The model under review builds one solid part; all positions refer to its coordinate system, in mm. Face numbers are marked on the shaded views. A direction names the side the tool comes from. Round coordinates to 2 decimals unless told otherwise and drop trailing zeros. Loops run counter-clockwise (first coordinate to the right, second up) from the corner with the lowest first, then second, coordinate; pieces in that order, holes last. Notation, with made-up numbers: M 1,79.5 L 27,79.5 A17 ccw 27,111.5 Z; hole C 87.25,20 d1. An arc over 180 degrees is marked long. Answer as a JSON object with one key per item and string values. Group by question number.
Item 1: Consider section A-A (x = 9.25). Give the boundary of the cut face in (y, z).
Item 2: Insertion check: P1, Ø0.5, axis at x = -3.5, z = -0.5, coming from the +Y side; P2, Ø1, axis at x = 11, z = 3, coming from the -Y side; P3, Ø2, axis at x = 1.5, z = -0.5, coming from the +Y side. Each pin has a flat end and moves straight along its axis. Give the tip position at first contact, or say it passes through.
Item 3: Tool access review of the marked faces 1 and 2: name each direction out of +Z, -Z, +X, -X, +Y, -Y from which nothing blocks a thin tool from reaching the whole face with its end or side.
Item 4: The part is to be moulded in two halves that separate along Z. For the marked faces 3 and 4, say which applies: +Z half, -Z half, draft (parallel to the pull), parting line (faces both ways), or undercut.
Item 5: To check wall thickness, follow line 1 (X direction, y = 1, z = 4.25); line 2 (X direction, y = 1.25, z = 1.75); line 3 (X direction, y = 2, z = -0.25). State the ranges of each line that lie inside material, in increasing order.
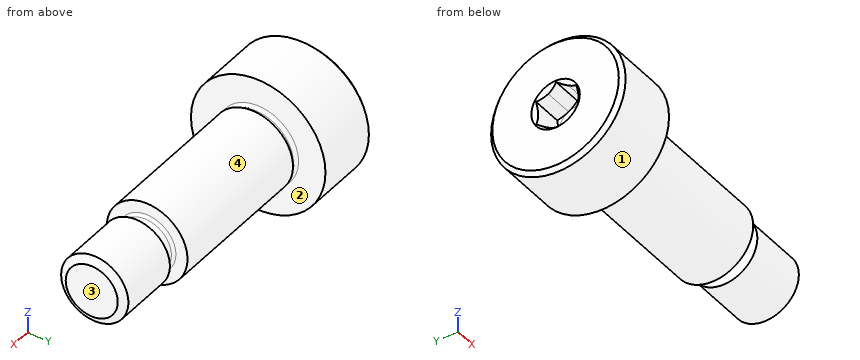
```python
from build123d import *

# Parameters (mm, degrees)
HEXEXTRUDE_START = -2.5000001
HEXEXTRUDE_DEPTH = 2.5000001


with BuildPart() as part:
    # Sketch2 → ScrewRevolve (revolve)
    with BuildSketch(Plane.XY, mode=Mode.PRIVATE) as screwrevolve_sk:
        with BuildLine():
            Line((18.02, 1.9345), (17.693508423, 2.5))
            Line((17.693508423, 2.5), (13.199474732, 2.5))
            Line((13.199474732, 2.5), (12.872983154, 1.9345))
            Line((12.872983154, 1.9345), (12.22, 1.9345))
            ThreePointArc((12.22, 1.9345), (12.078578644, 1.993078644), (12.02, 2.1345))
            Line((12.02, 2.1345), (12.02, 3))
            Line((12.02, 3), (0.6, 3))
            Line((0.6, 3), (0.3, 2.826794919))
            ThreePointArc((0.3, 2.826794919), (0.1, 2.826794919), (0, 3))
            Line((0, 3), (0, 5))
            Line((0, 5), (-4.7, 5))
            Line((-4.7, 5), (-5, 4.7))
            Line((-5, 4.7), (-5, 1.8))
            Line((-5, 1.8), (-4.7, 1.5))
            Line((-4.7, 1.5), (-2.5, 1.5))
            Line((-2.5, 1.5), (-1.598709071, 0))
            Line((-1.598709071, 0), (18.02, 0))
            Line((18.02, 0), (18.02, 1.9345))
        make_face()
    revolve(screwrevolve_sk.sketch.rotate(Axis((-1.598709071, 0, 0), (1, 0, 0)), 180), axis=Axis((-1.598709071, 0, 0), (1, 0, 0)))

    # HexExtrude: read off the stored shape, not the designer's step
    # HexExtrude outline → HexExtrude (cut)
    with BuildSketch(Plane.ZY.offset(5).offset(HEXEXTRUDE_START)):
        with BuildLine():
            Line((0, 1.5), (-0.866025404, 1.5))
            Line((-0.866025404, 1.5), (-1.299038105, 0.750000001))
            ThreePointArc((-1.299038105, 0.750000001), (-0.75, 1.299038106), (0, 1.5))
        make_face()
        with BuildLine():
            ThreePointArc((-1.299038107, -0.749999998), (-1.5, 2e-09), (-1.299038105, 0.750000001))
            Line((-1.299038105, 0.750000001), (-1.732050808, 0))
            Line((-1.732050808, 0), (-1.299038107, -0.749999998))
        make_face()
        with BuildLine():
            Line((0.866025404, 1.5), (0, 1.5))
            ThreePointArc((0, 1.5), (0.750000004, 1.299038103), (1.299038111, 0.749999991))
            Line((1.299038111, 0.749999991), (0.866025404, 1.5))
        make_face()
        with BuildLine():
            ThreePointArc((0, -1.5), (-0.750000001, -1.299038105), (-1.299038107, -0.749999998))
            Line((-1.299038107, -0.749999998), (-0.866025404, -1.5))
            Line((-0.866025404, -1.5), (0, -1.5))
        make_face()
        with BuildLine():
            Line((1.732050808, 0), (1.299038111, 0.749999991))
            ThreePointArc((1.299038111, 0.749999991), (1.5, -1e-09), (1.29903811, -0.749999993))
            Line((1.29903811, -0.749999993), (1.732050808, 0))
        make_face()
        with BuildLine():
            ThreePointArc((1.29903811, -0.749999993), (0.750000003, -1.299038104), (0, -1.5))
            Line((0, -1.5), (0.866025404, -1.5))
            Line((0.866025404, -1.5), (1.29903811, -0.749999993))
        make_face()
    extrude(amount=HEXEXTRUDE_DEPTH, mode=Mode.SUBTRACT)

    # HexExtrude 2 outline → HexExtrude 2 (revolve)
    with BuildSketch(Plane.YX):
        Polygon((1.732050808, -2.4999999), (1.5, -2.4999999), (1.732050809, -2.639430193), align=None)
    revolve(axis=Axis((0, 0, 0), (1, 0, 0)))


solid = part.part
```
Geometry results:
{
 "1": {"outline": "C 0,0 d6"},
 "2": {"P1": "stops at y = 4.99", "P2": "stops at y = -1.66", "P3": "stops at y = 3"},
 "3": {"face 1": "+X, -X", "face 2": "+X"},
 "4": {"face 3": "draft", "face 4": "parting line"},
 "5": {"line 1": "x = -5 to 0", "line 2": "x = -5 to 12.02, 13 to 17.9", "line 3": "x = -5 to 12.06, 12.92 to 17.97"}
}
